Model file for the job. Use its own axes, mm. A direction names the side the tool comes from. Round coordinates to 2 decimals unless told otherwise and drop trailing zeros. Order: outer loops, then holes, each group sorted by start corner. A loop starts at its lowest first (then second) coordinate and runs counter-clockwise, first axis right, second up. Notation, with made-up numbers: (21, 27.5) - (77, 27.5) arc R27 cw to (77, 61.5) - close; hole circle Ø11 at (62, -4). An arc over 180 degrees is marked (long way). Put each result on its own line as item: value. Start each with the question number.
Item 1: Pin check, flat tips, straight feed: pin 1 Ø1.5 at (x, y) = (-2, 90) entering from -Z; pin 2 Ø4 at (y, z) = (6.43, 6.43) entering from -X; pin 3 Ø0.9 at (x, z) = (-1, 35) entering from +Y. Stop position of each tip, or through.
Item 2: Probe probe 1 along Z at (x, y) = (-1, 6.43); probe 2 along Y at (x, z) = (-0.35, 55.5); probe 3 along Z at (x, y) = (-1.8, 91.5). List the from-to ranges inside material, lowest first.
Item 3: Saw through at A-A on y = 30. List the corners of the cut face in (x, z).
Item 4: Saw through at C-C on x = -0.85. List the corners of the cut face in (y, z).
Item 5: Saw through at B-B on z = 53.57. List the corners of the cut face in (x, y), plus the area to 3 significant figures.
Item 6: Saw through at D-D on y = 6.43. List the corners of the cut face in (x, z), plus the area to 3 significant figures.
Item 7: Which spindle directions (+Z, -Z, +X, -X, +Y, -Y) get a long thin tool onto all of the face, cutting with end or side? Do faces 1 (the face through (-2, 86, 37)), 2 (the face through (-1.52, 11.83, 35.72)). Say none if no direction does.
Item 8: Mould opens along Y. For faces 3 (the face through (-2, 68, 35)), 4 (the face through (-2, 0, 30)), 5 (the face through (-1.521, 56.068, 53.68)), 6 (the face through (-2, 86, 34)) say: pulls with the +Y half, pulls with the -Y half, needs draft (parallel to the pull), parting line crosses it, or undercut.
```python
from build123d import *

# Parameters (mm, degrees)
SKETCH2_W          = 3
SKETCH2_H          = 104
BASE_FLANGE1_DEPTH = 60
SKETCH4_R          = 2.5
SKETCH4_R_2        = 19.05
CUT_EXTRUDE2_DEPTH = 10
SKETCH5_W          = 3
SKETCH5_H          = 36
CUT_EXTRUDE4_DEPTH = 10


# Sheet-metal steps are written as plain solids
with BuildPart() as part:
    # Sketch2 → Base-Flange1 (new body)
    with BuildSketch(Plane.XY):
        with Locations((-1.5, 52)):
            Rectangle(SKETCH2_W, SKETCH2_H)
    extrude(amount=BASE_FLANGE1_DEPTH)

    # Sketch4 → Cut-Extrude2 (cut)
    with BuildSketch(Plane.ZY.offset(3)):
        with Locations(Location((6.43, 6.43, 0), (0, 0, 270))):
            Circle(SKETCH4_R)
        with Locations(Location((30, 30, 0), (0, 0, 270))):
            Circle(SKETCH4_R_2)
        with Locations(Location((6.43, 53.57, 0), (0, 0, 270))):
            Circle(SKETCH4_R)
        with Locations(Location((53.57, 6.43, 0), (0, 0, 270))):
            Circle(SKETCH4_R)
        with Locations(Location((53.57, 53.57, 0), (0, 0, 270))):
            Circle(SKETCH4_R)
    extrude(amount=-CUT_EXTRUDE2_DEPTH, mode=Mode.SUBTRACT)

    # Sketch5 → Cut-Extrude4 (cut)
    with BuildSketch(Plane.ZY.offset(3)):
        with Locations((35.5, 86)):
            Rectangle(SKETCH5_W, SKETCH5_H)
    extrude(amount=-CUT_EXTRUDE4_DEPTH, mode=Mode.SUBTRACT)


solid = part.part
```
Results found:
1. pin 1: stops at z = 0
1. pin 2: passes through
1. pin 3: stops at y = 68
2. probe 1: z = 0 to 3.93, 8.93 to 51.07, 56.07 to 60
2. probe 2: y = 0 to 4.84, 8.02 to 51.98, 55.16 to 104
2. probe 3: z = 0 to 34, 37 to 60
3. outline: (-3, 0) - (0, 0) - (0, 10.95) - (-3, 10.95) - close; (-3, 49.05) - (0, 49.05) - (0, 60) - (-3, 60) - close
4. outline: (0, 0) - (104, 0) - (104, 34) - (68, 34) - (68, 37) - (104, 37) - (104, 60) - (0, 60) - close; hole circle Ø5 at (6.43, 6.43); hole circle Ø5 at (6.43, 53.57); hole circle Ø38.1 at (30, 30); hole circle Ø5 at (53.57, 6.43); hole circle Ø5 at (53.57, 53.57)
5. outline: (-3, 0) - (0, 0) - (0, 3.93) - (-3, 3.93) - close; (-3, 8.93) - (0, 8.93) - (0, 51.07) - (-3, 51.07) - close; (-3, 56.07) - (0, 56.07) - (0, 104) - (-3, 104) - close
5. area: 282 mm²
6. outline: (-3, 0) - (0, 0) - (0, 3.93) - (-3, 3.93) - close; (-3, 8.93) - (0, 8.93) - (0, 51.07) - (-3, 51.07) - close; (-3, 56.07) - (0, 56.07) - (0, 60) - (-3, 60) - close
6. area: 150 mm²
7. face 1: +X, -X, +Y
7. face 2: +X, -X
8. face 3: pulls with the +Y half
8. face 4: pulls with the -Y half
8. face 5: undercut
8. face 6: needs draft
